from build123d import *

# Parameters (mm, degrees)
F1_DEPTH      = 25
F2_W          = 38.0999911882
F2_H          = 25
F3_DEPTH      = 29.0380437433
F5_DEPTH      = 11.6510001
F5_DEPTH_BACK = 11.6510001


with BuildPart() as f1:
    # F0 (on Front) → F1 (new body)
    with BuildSketch(Plane.XZ):
        with BuildLine():
            ThreePointArc((-19.0499955941, 0.0129562567), (0, 19.05), (19.0499955941, 0.0129562567))
            Line((19.0499955941, 0.0129562567), (19.0499955941, 29.05))
            Line((19.0499955941, 29.05), (-19.0499955941, 29.05))
            Line((-19.0499955941, 29.05), (-19.0499955941, 0.0129562567))
        make_face()
    extrude(amount=F1_DEPTH)

    # F2 (on face) → F3 (cut, through all)
    with BuildSketch(Plane.XY.offset(29.05)):
        with Locations((0, -12.5)):
            Rectangle(F2_W, F2_H)
        with BuildLine():
            ThreePointArc((-11.65, -15.9987397492), (0, -4.3487397492), (11.65, -15.9987397492))
            Line((11.65, -15.9987397492), (9.6499996489, -15.9987397492))
            ThreePointArc((9.6499996489, -15.9987397492), (0, -6.3487401003), (-9.6499996489, -15.9987397492))
            Line((-9.6499996489, -15.9987397492), (-11.65, -15.9987397492))
        make_face(mode=Mode.SUBTRACT)
    extrude(amount=-F3_DEPTH, mode=Mode.SUBTRACT)

    # F4 (on Right) → F5 (cut, two sides)
    with BuildSketch(Plane.YZ) as f5_sk:
        with BuildLine():
            Line((-15.9987397492, 29.05), (-15.9987397492, 18.0724914994))
            add(Edge.make_bspline(
                [(-15.9987397492, 18.0724914994), (-13.4661328048, 22.3090033978), (-8.5014579818, 28.4231342375), (-4.3487397492, 29.05)],
                knots=[0, 0, 0, 0, 16.0071294391, 16.0071294391, 16.0071294391, 16.0071294391], degree=3))
            Line((-4.3487397492, 29.05), (-15.9987397492, 29.05))
        make_face()
    extrude(amount=-F5_DEPTH, mode=Mode.SUBTRACT)
    extrude(f5_sk.sketch, amount=F5_DEPTH_BACK, mode=Mode.SUBTRACT)


solid = f1.part
Check sheet for the modelled part. Datum: model origin and axes. Units: mm. Round coordinates to 2 decimals unless told otherwise and drop trailing zeros. One line per item, written item: value. Start each with the question number.
1. Gauge pin test, flat ends, axial feed: P1, Ø1, axis at x = -8, z = 18.5, coming from the -Y side; P2, Ø4, axis at x = -8.5, y = -14.5, coming from the -Z side; P3, Ø5, axis at y = -13.5, z = 26, coming from the +X side. Record the tip position at first contact, or that the pin passes through.
2. Scan lines: line 1 along X through (y, z) = (-11.5, 21.5); line 2 along X through (y, z) = (-8.25, 19); line 3 along Z through (x, y) = (-1, -4.75). Record each from-to range of solid material in increasing order.
3. Release check for a two-part mould opening along X. For faces 1 (the cylindrical face through (-0.26, -4.35, 22.16)), 2 (the flat face through (11, -15.999, 17)), 3 (the cylindrical face through (1.796, -6.261, 18.965)) record: released by +X, released by -X, zero draft, split by the parting line, or undercut.
Results found:
1. P1: y = -11.43
1. P2: z = 15.9
1. P3: through
2. line 1: -10.75 to -8.54, 8.54 to 10.75
2. line 2: -8.7 to -5.75, 5.75 to 8.7
2. line 3: 19.02 to 28.97
3. face 1: split by the parting line
3. face 2: zero draft
3. face 3: undercut
